Read the model definition and answer for the solid it produces. Units are mm, in the model's axes. Give positions to 0.01 mm unless a question says otherwise; leave off trailing zeros. Write each loop counter-clockwise with the first axis right and the second up, starting at its lowest first coordinate (ties: lowest second). Pieces come first, ordered by that corner, then holes. Notation, with made-up numbers: M 41.5,68 L 56.5,68 A26 ccw 56.5,100 Z; hole C 16.25,27.25 d9. An arc over 180 degrees is marked long. Answer as CSV lines item,"result". Start each with the question number.
Autodesk Inventor part; units mm, degrees
ref_plane "YZ Plane" through (0, 0, 0) normal (1, 0, 0) x (0, 1, 0)
ref_plane "XZ Plane" through (0, 0, 0) normal (0, 1, 0) x (-1, 0, 0)
ref_plane "XY Plane" through (0, 0, 0) normal (0, 0, 1) x (1, 0, 0)
sketch "Sketch1" plane through (0, 0, 0) normal (0, 0, 1) x (1, 0, 0)
  line L0 (0, 0) -> (0, 6.35) construction
  line L1 (3.6591, 6.35) -> (7.3288, 0.0061)
  line L2 (7.3288, 0.0061) -> (3.6697, -6.3439)
  line L3 (3.6697, -6.3439) -> (-3.6591, -6.35)
  line L4 (-3.6591, -6.35) -> (-7.3288, -0.0061)
  line L5 (-7.3288, -0.0061) -> (-3.6697, 6.3439)
  line L6 (-3.6697, 6.3439) -> (3.6591, 6.35)
  dimension "d0" = 6.35
extrude "Extrusion1" add sketch "Sketch1" along normal blind 482.6
properties part number "Hex Shaft ARm"
1. Find section B-B on y = 4.25. Determine the outline of the cut face in (x, z).
2. Given pin 1 (1 mm diameter, centred on y = -3.5, z = 411.5, fed in from -X); pin 2 (1.5 mm diameter, centred on y = 2.5, z = 388.5, fed in from +X); pin 3 (2 mm diameter, centred on y = -4.5, z = 266.5, fed in from +X), each flat-ended and moving along its own axis, determine where each tip first touches the part or whether it passes through.
3. Find section A-A on z = 120. Determine the outline of the cut face in (x, y), then the cut area to 3 significant figures.
4. Find the intervals of material crossed by line 1 (Y direction, x = -0.75, z = 233.5); line 2 (X direction, y = -1.75, z = 358); line 3 (Y direction, x = -5.25, z = 411), in increasing order. Write a range as [from, to].
Computed:
1,outline,"M -4.88,0 L 4.87,0 L 4.87,482.6 L -4.88,482.6 Z"
2,pin 1,"stops at x = -5.6"
2,pin 2,"stops at x = 6.32"
2,pin 3,"stops at x = 5.31"
3,outline,"M -7.33,-0.01 L -3.66,-6.35 L 3.67,-6.34 L 7.33,0.01 L 3.66,6.35 L -3.67,6.34 Z"
3,area,"140 mm^2"
4,line 1,"y = [-6.35, 6.35]"
4,line 2,"x = [-6.32, 6.32]"
4,line 3,"y = [-3.6, 3.6]"
